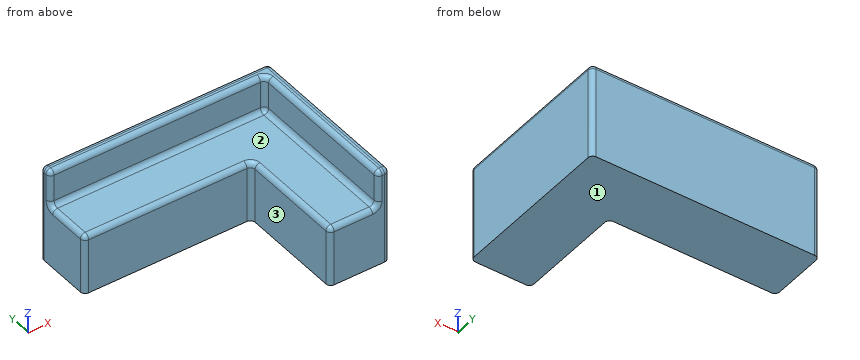
```python
from build123d import *

# Parameters (mm, degrees)
F1_DEPTH = 101.6
F2_DEPTH = 63.5
F3_R     = 5.08


with BuildPart() as f1:
    # F0 (on Top) → F1 (new body)
    with BuildSketch(Plane.XY):
        Polygon((28.1707099802, 104.9363430021), (-200.4292900198, 104.9363430021), (-200.4292900198, 92.2363430021), (28.1707099802, 92.2363430021), (28.1707099802, -72.8636569979), (40.8707099802, -72.8636569979), (40.8707099802, 41.4363430021), (40.8707099802, 92.2363430021), (40.8707099802, 104.9363430021), align=None)
    extrude(amount=F1_DEPTH)

    # F0 (on Top) → F2 (join)
    with BuildSketch(Plane.XY):
        Polygon((28.1707099802, 104.9363430021), (-200.4292900198, 104.9363430021), (-200.4292900198, 92.2363430021), (28.1707099802, 92.2363430021), (28.1707099802, -72.8636569979), (40.8707099802, -72.8636569979), (40.8707099802, 41.4363430021), (40.8707099802, 92.2363430021), (40.8707099802, 104.9363430021), align=None)
        Polygon((28.1707099802, 92.2363430021), (-200.4292900198, 92.2363430021), (-200.4292900198, 41.4363430021), (-22.6292900198, 41.4363430021), (-22.6292900198, -72.8636569979), (28.1707099802, -72.8636569979), align=None)
    extrude(amount=F2_DEPTH)

    # F3
    f3_edges = [f1.edges().sort_by_distance(p)[0] for p in [
        (28.17071, 9.686343, 101.6),
        (-86.12929, 92.236343, 101.6),
        (28.17071, 92.236343, 82.55),
        (28.17071, 9.686343, 63.5),
        (28.17071, -72.863657, 82.55),
        (-200.42929, 92.236343, 82.55),
        (-86.12929, 92.236343, 63.5),
        (2.77071, -72.863657, 63.5),
        (-22.62929, -15.713657, 63.5),
        (-111.52929, 41.436343, 63.5),
        (-200.42929, 66.836343, 63.5),
        (-22.62929, 41.436343, 31.75),
        (-200.42929, 41.436343, 31.75),
        (-79.77929, 104.936343, 101.6),
        (40.87071, 16.036343, 101.6),
        (34.52071, -72.863657, 101.6),
        (-200.42929, 98.586343, 101.6),
        (-22.62929, -72.863657, 31.75),
        (-200.42929, 104.936343, 50.8),
        (40.87071, -72.863657, 50.8),
        (40.87071, 104.936343, 50.8),
    ]]
    fillet(f3_edges, radius=F3_R)


solid = f1.part
```
Geometry check sheet. Reference: the model listing, model coordinates, mm. Face numbers are marked on the shaded views. A direction names the side the tool comes from. Round coordinates to 2 decimals unless told otherwise and drop trailing zeros. Order: outer loops, then holes, each group sorted by start corner. A loop starts at its lowest first (then second) coordinate and runs counter-clockwise, first axis right, second up. Notation, with made-up numbers: (-27.75, 71.5) - (15.25, 71.5) arc R33 cw to (15.25, 101.5) - close; hole circle Ø10 at (-23.75, -35.5). An arc over 180 degrees is marked (long way). Use a Markdown table: item, result. Add a question column.
1) Set-up check for the marked faces 1, 2 and 3: record each of +Z, -Z, +X, -X, +Y, -Y from which the full face is reachable in a straight line by a thin tool's end or side.
2) Section check A-A (y = 64). Record the cut outline in (x, z).
3) Thickness scan on line 1 along X through (y, z) = (-28, 44); line 2 along Y through (x, z) = (-95, 27); line 3 along X through (y, z) = (58, 80). Record the ranges inside material, lowest first.
4) Section check C-C (x = -109). Record the cut outline in (y, z).
5) Section check B-B (z = 86). Record the cut outline in (x, y), then the cut area to 3 significant figures.
6) Gauge pin test, flat ends, axial feed: P1, Ø8.5, axis at y = 30, z = 88, coming from the -X side; P2, Ø1, axis at x = -14.5, y = 13.5, coming from the +Z side; P3, Ø5, axis at x = 15.5, z = 68, coming from the -Y side; P4, Ø2, axis at x = -91, y = 41, coming from the -Z side. Record the tip position at first contact, or that the pin passes through.
7) Section check D-D (z = 33). Record the cut outline in (x, y), then the cut area to 3 significant figures.
Established:
| question | item | result |
|---|---|---|
| 1 | face 1 | -Z, +X, -X, +Y, -Y |
| 1 | face 2 | +Z, -X, -Y |
| 1 | face 3 | +Z, -Z, -X, -Y |
| 2 | outline | (-200.43, 0) - (40.87, 0) - (40.87, 96.52) arc R5.08 ccw to (35.79, 101.6) - (33.25, 101.6) arc R5.08 ccw to (28.17, 96.52) - (28.17, 68.58) arc R5.08 cw to (23.09, 63.5) - (-195.35, 63.5) arc R5.08 ccw to (-200.43, 58.42) - close |
| 3 | line 1 | -22.63 to 40.87 |
| 3 | line 2 | 41.44 to 104.94 |
| 3 | line 3 | 28.17 to 40.87 |
| 4 | outline | (41.44, 0) - (104.94, 0) - (104.94, 96.52) arc R5.08 ccw to (99.86, 101.6) - (97.32, 101.6) arc R5.08 ccw to (92.24, 96.52) - (92.24, 68.58) arc R5.08 cw to (87.16, 63.5) - (46.52, 63.5) arc R5.08 ccw to (41.44, 58.42) - close |
| 5 | outline | (-200.43, 97.32) arc R5.08 ccw to (-195.35, 92.24) - (23.09, 92.24) arc R5.08 cw to (28.17, 87.16) - (28.17, -67.78) arc R5.08 ccw to (33.25, -72.86) - (35.79, -72.86) arc R5.08 ccw to (40.87, -67.78) - (40.87, 99.86) arc R5.08 ccw to (35.79, 104.94) - (-195.35, 104.94) arc R5.08 ccw to (-200.43, 99.86) - close |
| 5 | area | 5,140 mm2 |
| 6 | P1 | x = 28.17 |
| 6 | P2 | z = 63.5 |
| 6 | P3 | y = 91.2 |
| 6 | P4 | z = 0 |
| 7 | outline | (-200.43, 46.52) arc R5.08 ccw to (-195.35, 41.44) - (-27.71, 41.44) arc R5.08 cw to (-22.63, 36.36) - (-22.63, -67.78) arc R5.08 ccw to (-17.55, -72.86) - (35.79, -72.86) arc R5.08 ccw to (40.87, -67.78) - (40.87, 99.86) arc R5.08 ccw to (35.79, 104.94) - (-195.35, 104.94) arc R5.08 ccw to (-200.43, 99.86) - close |
| 7 | area | 22,600 mm2 |
